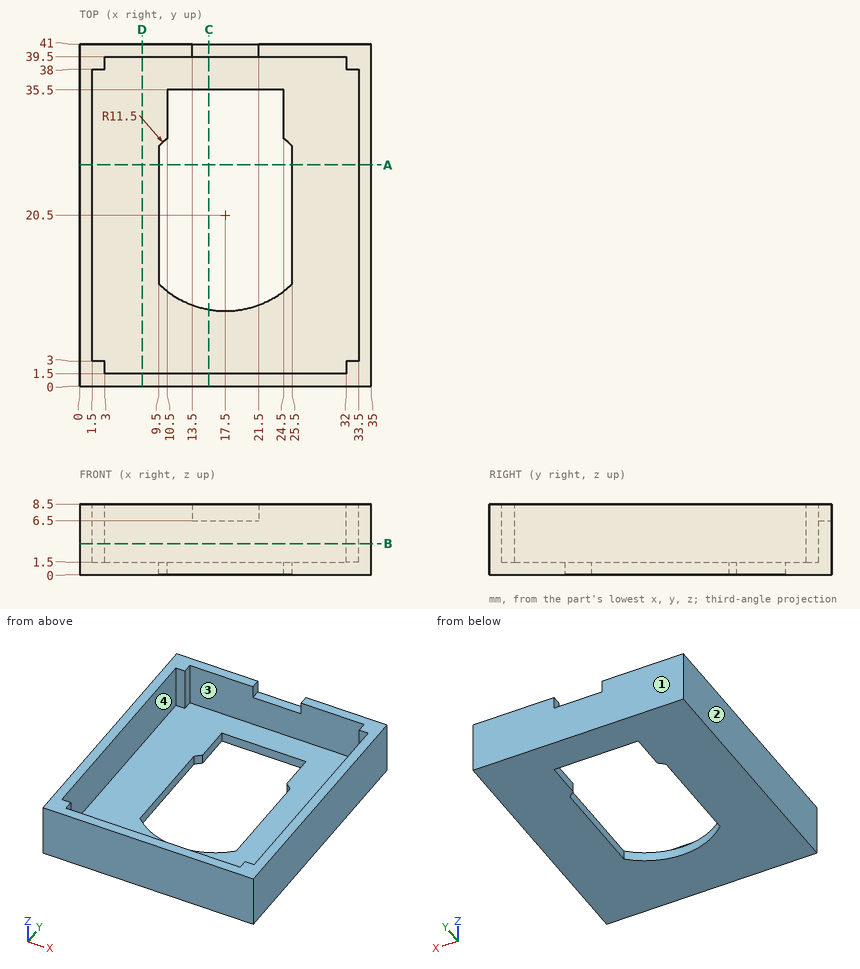
Study the drawing (mm; zero at the part's minimum x, y, z) and answer. Coordinates: 2 decimals unless noted, no trailing zeros. Loops run counter-clockwise (first coordinate to the right, second up) from the corner with the lowest first, then second, coordinate; pieces in that order, holes last. Notation, with made-up numbers: M 48,-3.5 L 83,-3.5 A17 cw 83,1.5 Z; hole C 33.5,-19 d7. An arc over 180 degrees is marked long. Answer in a Markdown table with one row per item.
1) Determine the mould class of the marked faces 1, 2, 3 and 4 for opening direction Y: released by +Y, released by -Y, zero draft, split by the parting line, or undercut.
Answers below:
| item | result |
|---|---|
| face 1 | released by +Y |
| face 2 | zero draft |
| face 3 | undercut |
| face 4 | undercut |
2) Given pin 1 (16 mm diameter, centred on x = 21.5, y = 16.5, fed in from +Z); pin 2 (1.6 mm diameter, centred on x = 17, y = 40.5, fed in from +Z); pin 3 (4 mm diameter, centred on x = 22, y = 20, fed in from -Z), each flat-ended and moving along its own axis, determine where each tip first touches the part or whether it passes through.
Answers below:
| item | result |
|---|---|
| pin 1 | z = 1.5 |
| pin 2 | z = 6.5 |
| pin 3 | through |
3) Find section D-D (x = 7.5). Determine the outline of the cut face in (y, z).
Answers below:
| item | result |
|---|---|
| outline | M 0,0 L 41,0 L 41,8.5 L 39.5,8.5 L 39.5,1.5 L 1.5,1.5 L 1.5,8.5 L 0,8.5 Z |
4) Find section C-C (x = 15.5). Determine the outline of the cut face in (y, z).
Answers below:
| item | result |
|---|---|
| outline | M 0,0 L 9.18,0 L 9.18,1.5 L 1.5,1.5 L 1.5,8.5 L 0,8.5 Z; M 35.5,0 L 41,0 L 41,6.5 L 39.5,6.5 L 39.5,1.5 L 35.5,1.5 Z |
5) Find section A-A (y = 26.5). Determine the outline of the cut face in (x, z).
Answers below:
| item | result |
|---|---|
| outline | M 0,0 L 9.5,0 L 9.5,1.5 L 1.5,1.5 L 1.5,8.5 L 0,8.5 Z; M 25.5,0 L 35,0 L 35,8.5 L 33.5,8.5 L 33.5,1.5 L 25.5,1.5 Z |
6) Find the intervals of material crossed by probe 1 along Y at (x, z) = (7, 4.75); probe 2 along X at (y, z) = (32.5, 5); probe 3 along X at (y, z) = (32.5, 1), in increasing order.
Answers below:
| item | result |
|---|---|
| probe 1 | 0 to 1.5, 39.5 to 41 |
| probe 2 | 0 to 1.5, 33.5 to 35 |
| probe 3 | 0 to 10.5, 24.5 to 35 |
7) Find section B-B (z = 3.75). Determine the outline of the cut face in (x, y), then the cut area to 3 significant figures.
Answers below:
| item | result |
|---|---|
| outline | M 0,0 L 35,0 L 35,41 L 0,41 Z; hole M 1.5,3 L 3,3 L 3,1.5 L 32,1.5 L 32,3 L 33.5,3 L 33.5,38 L 32,38 L 32,39.5 L 3,39.5 L 3,38 L 1.5,38 Z |
| area | 228 mm^2 |
